Can you work these out from the drawing? Everything is in mm from the part's minimum corner. A direction names the side the tool comes from. Give positions to 0.01 mm unless a question says otherwise; leave off trailing zeros. Order: outer loops, then holes, each group sorted by start corner. A loop starts at its lowest first (then second) coordinate and runs counter-clockwise, first axis right, second up. Notation, with made-up numbers: M 40.5,-28 L 61.5,-28 A26 cw 61.5,8 Z; hole C -1,-28 d8. An arc over 180 degrees is marked long. Answer in a Markdown table with one row per item. Add a question column.
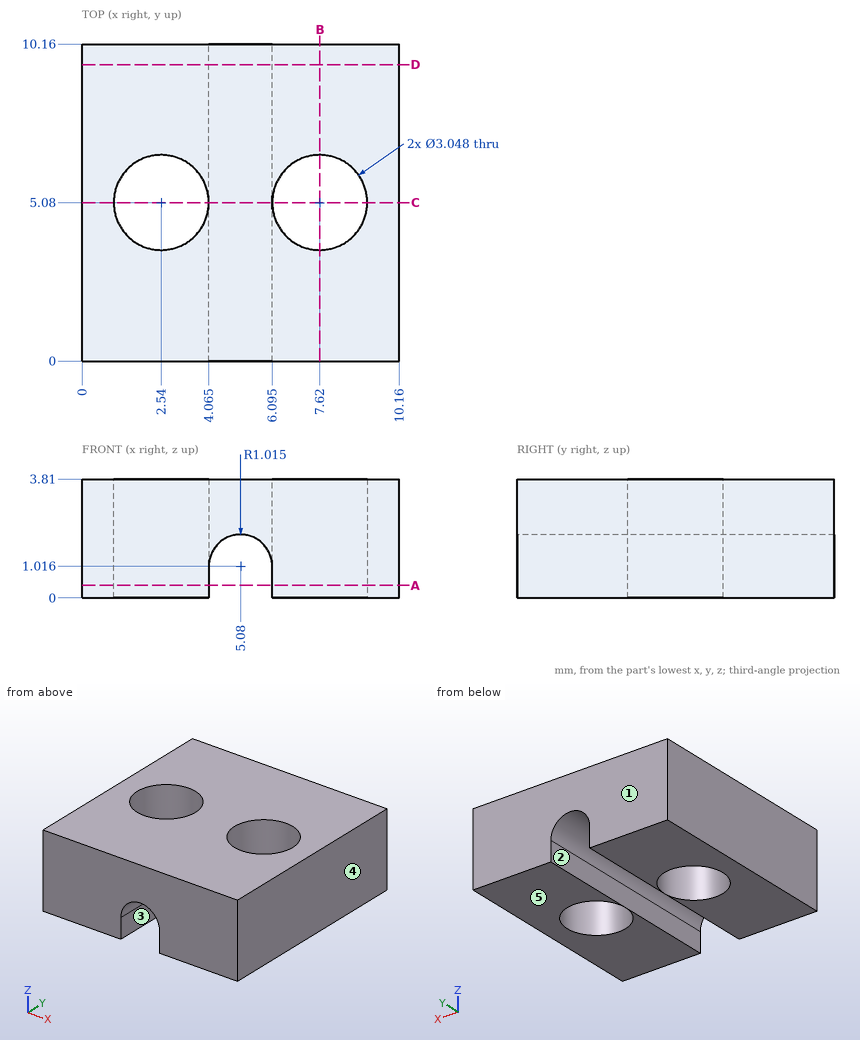
1. Suppose I cut it at A-A on z = 0.4. List the corners of the cut face in (x, y) for me (1 decimal).
2. Suppose I cut it at B-B on x = 7.62. List the corners of the cut face in (y, z) for me.
3. Thinking about a two-plate mould opening in X: for the marked faces 3, 4 and 5, which applies, pulls with the +X half, pulls with the -X half, needs draft (parallel to the pull), parting line crosses it, or undercut?
4. For the marked faces 1 and 2, which set-ups out of +Z, -Z, +X, -X, +Y, -Y let a thin tool reach every point of the face, with its end or its side?
5. Will this pin go through, and if not, where does the flat tip stop? P1, Ø2.5, axis at x = 7.62, y = 5.08, coming from the +Z side.
6. Suppose I cut it at D-D on y = 9.5. List the corners of the cut face in (x, z) for me (1 decimal).
7. Suppose I cut it at C-C on y = 5.08. Count the separate pieces of the cut face and the enclosed holes in it, plus the area to 3 significant figures.
8. If I drill on line 1 along Y through (x, z) = (2.54, 2.5); line 2 along X through (y, z) = (7, 1.05); line 3 along Z through (x, y) = (5, 2), over which ranges is the centre line in solid material (lowest first)? Write a range as [from, to].
Findings below:
| question | item | result |
|---|---|---|
| 1 | outline | M 0,0 L 4.1,0 L 4.1,10.2 L 0,10.2 Z; M 6.1,0 L 10.2,0 L 10.2,10.2 L 6.1,10.2 Z; hole C 2.5,5.1 d3; hole C 7.6,5.1 d3 |
| 2 | outline | M 0,0 L 3.56,0 L 3.56,3.81 L 0,3.81 Z; M 6.6,0 L 10.16,0 L 10.16,3.81 L 6.6,3.81 Z |
| 3 | face 3 | undercut |
| 3 | face 4 | pulls with the +X half |
| 3 | face 5 | needs draft |
| 4 | face 1 | +Z, -Z, +X, -X, +Y |
| 4 | face 2 | -Z, +Y, -Y |
| 5 | P1 | through |
| 6 | outline | M 0,0 L 4.1,0 L 4.1,1 A1 cw 6.1,1 L 6.1,0 L 10.2,0 L 10.2,3.8 L 0,3.8 Z |
| 7 | separate pieces | 3 |
| 7 | enclosed holes | 0 |
| 7 | area | 11.8 mm2 |
| 8 | line 1 | [0, 3.56], [6.6, 10.16] |
| 8 | line 2 | [0, 4.07], [6.09, 10.16] |
| 8 | line 3 | [2.03, 3.81] |
